Here's the drawing with two shaded views (mm, measured from the low corner). I have some questions. A direction names the side the tool comes from. Round coordinates to 2 decimals unless told otherwise and drop trailing zeros. Loops run counter-clockwise (first coordinate to the right, second up) from the corner with the lowest first, then second, coordinate; pieces in that order, holes last. Notation, with made-up numbers: (7.5, 37) -> (50.5, 37) arc R30 cw to (50.5, 64) -> close; hole circle Ø7 at (82.25, -6.5). An arc over 180 degrees is marked (long way). Write each question's results on one line, items separated by ' | '. Start each with the question number.
1) For P1, Ø12.5, axis at x = 26, y = 23.5, coming from the -Z side; P2, Ø6, axis at y = 9.5, z = 9.5, coming from the +X side; P3, Ø10.5, axis at x = 31.5, y = 6.5, coming from the +Z side, each with a flat end and sliding along its axis, tell me the tip position at first contact or that it passes through.
2) If I drill on probe 1 along Y at (x, z) = (54, 37) (1 decimal); probe 2 along Y at (x, z) = (57, 9.5); probe 3 along Z at (x, y) = (35.5, 11.5), over which ranges is the centre line in solid material (lowest first)?
3) Imagine slicing it at D-D, the plane y = 11. List the corners of the cut face in (x, z) for me.
4) Which directions (+Z, -Z, +X, -X, +Y, -Y) give clear straight access to the entire face, cutting with the end or side of a thin tool? Please do the marked faces 1, 2, 3, 4 and 5.
5) Imagine slicing it at A-A, the plane z = 29. List the corners of the cut face in (x, y) for me (1 decimal).
6) Imagine slicing it at C-C, the plane z = 8. List the corners of the cut face in (x, y) for me.
7) We'd pull the mould along Y, two halves only. Please class the marked faces 6, 7 and 8: pulls with the +Y half, pulls with the -Y half, needs draft (parallel to the pull), parting line crosses it, or undercut.
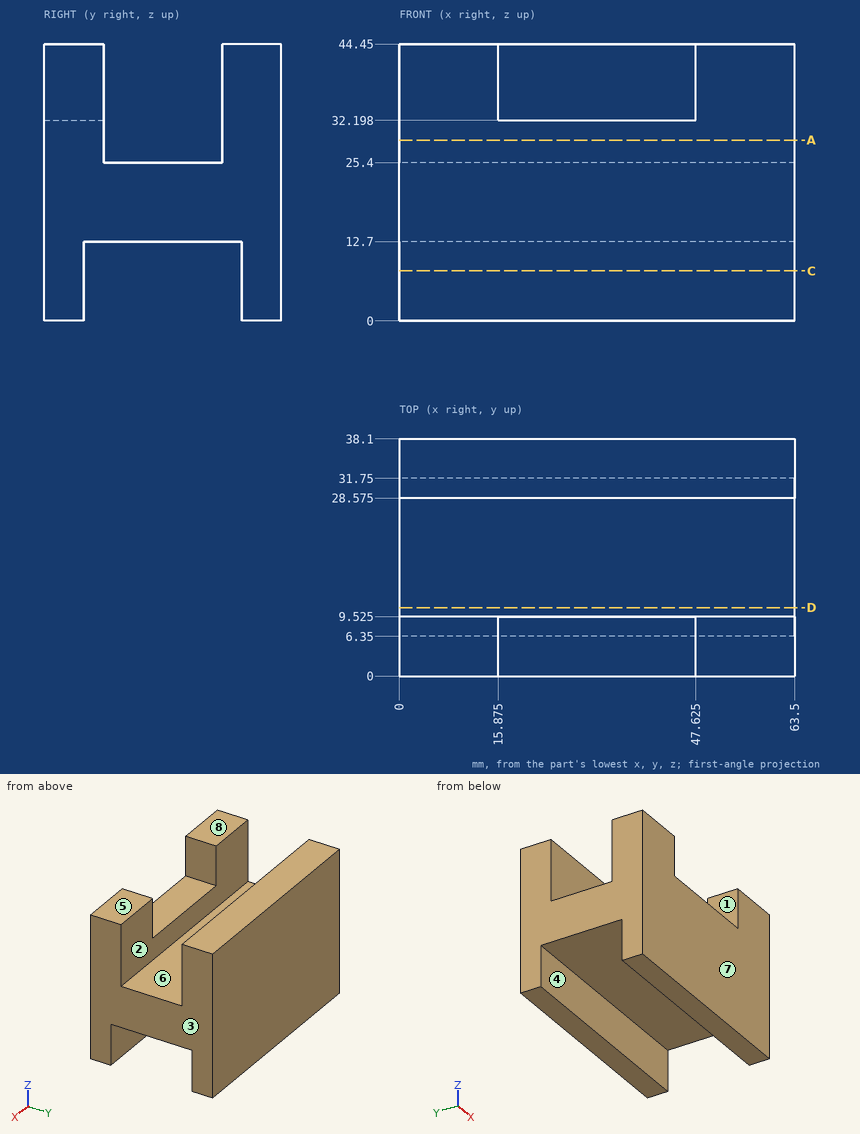
Checked values:
1) P1: z = 12.7 | P2: through | P3: z = 32.2
2) probe 1: 0 to 9.5, 28.6 to 38.1 | probe 2: 0 to 6.35, 31.75 to 38.1 | probe 3: 12.7 to 25.4
3) outline: (0, 12.7) -> (63.5, 12.7) -> (63.5, 25.4) -> (0, 25.4) -> close
4) face 1: +Z, -Y | face 2: +Z, +X, -X | face 3: +Z, -Z, +X, +Y, -Y | face 4: -Z, +X, -X | face 5: +Z, +X, -X, +Y, -Y
5) outline: (0, 0) -> (63.5, 0) -> (63.5, 9.5) -> (0, 9.5) -> close; (0, 28.6) -> (63.5, 28.6) -> (63.5, 38.1) -> (0, 38.1) -> close
6) outline: (0, 0) -> (63.5, 0) -> (63.5, 6.35) -> (0, 6.35) -> close; (0, 31.75) -> (63.5, 31.75) -> (63.5, 38.1) -> (0, 38.1) -> close
7) face 6: undercut | face 7: pulls with the -Y half | face 8: needs draft
